Geometry check sheet. Reference: the model listing, model coordinates, mm. A direction names the side the tool comes from. Round coordinates to 2 decimals unless told otherwise and drop trailing zeros. Write each loop counter-clockwise with the first axis right and the second up, starting at its lowest first coordinate (ties: lowest second). Pieces come first, ordered by that corner, then holes. Notation, with made-up numbers: M 81,35.25 L 85,35.25 A18 ccw 85,58.25 Z; hole C 10.5,-11.75 d5. An arc over 180 degrees is marked long. Use a Markdown table: item, result.
```python
from build123d import *

# Parameters (mm, degrees)
CYLINDER052_R             = 6.25
CYLINDER052_DEPTH         = 17
CYLINDER051_R             = 2.1
CYLINDER051_DEPTH         = 10
EXTRUDE014_DEPTH          = 10
EXTRUDE016_DEPTH          = 14
EXTRUDE015_DEPTH          = 4
BOX021_W                  = 47
BOX021_H                  = 26
BOX021_DEPTH              = 4
CYLINDER044_R             = 4
CYLINDER044_DEPTH         = 4
BOX014_W                  = 13
BOX014_H                  = 8
BOX014_DEPTH              = 4
FUSION015_PLACEMENT_ANGLE = 180
CYLINDER039_R             = 1.6
CYLINDER039_DEPTH         = 15
CYLINDER043_R             = 3.7
CYLINDER043_DEPTH         = 10
CYLINDER045_R             = 7.5
CYLINDER045_DEPTH         = 6
CYLINDER042_R             = 9.6
CYLINDER042_DEPTH         = 6
BOX012_W                  = 26
BOX012_H                  = 42
BOX012_DEPTH              = 1
BOX013_W                  = 47
BOX013_H                  = 10
BOX013_DEPTH              = 37


with BuildPart() as cylinder052:
    # Cylinder052 → Cylinder052 (new body)
    with BuildSketch(Plane.XY.offset(10)):
        Circle(CYLINDER052_R)
    extrude(amount=CYLINDER052_DEPTH)


with BuildPart() as fusion022:
    # Cylinder051 → Cylinder051 (new body)
    with BuildSketch(Plane.XY):
        Circle(CYLINDER051_R)
    extrude(amount=CYLINDER051_DEPTH)

    # Fusion022: union Cylinder052
    add(cylinder052.part)


with BuildPart() as fusion022_1:
    # Fusion022 placement: moved
    add(fusion022.part.moved(Location((12, 12, -6))))


with BuildPart() as extrude014:
    # Sketch010 → Extrude014 (new body)
    with BuildSketch(Plane.XY):
        with BuildLine():
            ThreePointArc((35.736492, 10), (36.2, 15), (35.736492, 20))
            ThreePointArc((35.736492, 20), (33.490746, 22.111711), (31.244999, 20))
            ThreePointArc((31.244999, 10), (31.8, 15), (31.244999, 20))
            ThreePointArc((31.244999, 10), (33.490746, 7.888289), (35.736492, 10))
        make_face()
    extrude(amount=-EXTRUDE014_DEPTH)


with BuildPart() as extrude014_1:
    # Extrude014 placement: moved
    add(extrude014.part.moved(Location((2, -3, 8))))


with BuildPart() as extrude016:
    # Sketch015 → Extrude016 (new body)
    with BuildSketch(Plane.YZ):
        Polygon((0, 4), (26, 4), (26, 23), align=None)
    extrude(amount=EXTRUDE016_DEPTH)


with BuildPart() as extrude015:
    # Sketch014 → Extrude015 (new body)
    with BuildSketch(Plane.YZ):
        Polygon((0, 4), (26, 4), (26, 37), align=None)
    extrude(amount=EXTRUDE015_DEPTH)


with BuildPart() as extrude015_1:
    # Extrude015 placement: moved
    add(extrude015.part.moved(Location((43, 0, 0))))


with BuildPart() as box021:
    # Box021 → Box021 (new body)
    with BuildSketch(Plane.XY):
        with Locations((23.5, 13)):
            Rectangle(BOX021_W, BOX021_H)
    extrude(amount=BOX021_DEPTH)


with BuildPart() as cylinder044:
    # Cylinder044 → Cylinder044 (new body)
    with BuildSketch(Plane(origin=(9, 11, -8), x_dir=(1, 0, 0), z_dir=(0, 0, 1))):
        Circle(CYLINDER044_R)
    extrude(amount=CYLINDER044_DEPTH)


with BuildPart() as fusion015:
    # Box014 → Box014 (new body)
    with BuildSketch(Plane(origin=(9, 7, -8), x_dir=(1, 0, 0), z_dir=(0, 0, 1))):
        with Locations((6.5, 4)):
            Rectangle(BOX014_W, BOX014_H)
    extrude(amount=BOX014_DEPTH)

    # Fusion015: union Cylinder044
    add(cylinder044.part)


with BuildPart() as fusion015_1:
    # Fusion015 placement: moved
    add(fusion015.part.moved(Location((13, 42, 21))).rotate(Axis((13, 42, 21), (0, 0, 1)), FUSION015_PLACEMENT_ANGLE))


with BuildPart() as cylinder039:
    # Cylinder039 → Cylinder039 (new body)
    with BuildSketch(Plane.XY):
        Circle(CYLINDER039_R)
    extrude(amount=CYLINDER039_DEPTH)


with BuildPart() as fusion016:
    # Cone002 → Cone002 (revolve)
    with BuildSketch(Plane(origin=(0, 0, 15), x_dir=(1, 0, 0), z_dir=(0, -1, 0))):
        Polygon((0, 0), (1.6, 0), (3, 3.5), (0, 3.5), align=None)
    revolve(axis=Axis((0, 0, 15), (0, 0, 1)))

    # Fusion016: union Cylinder039
    add(cylinder039.part)


with BuildPart() as fusion016_1:
    # Fusion016 placement: moved
    add(fusion016.part.moved(Location((4, 31, 13.5))))


with BuildPart() as cylinder043:
    # Cylinder043 → Cylinder043 (new body)
    with BuildSketch(Plane(origin=(4, 31, 32), x_dir=(1, 0, 0), z_dir=(0, 0, 1))):
        Circle(CYLINDER043_R)
    extrude(amount=CYLINDER043_DEPTH)


with BuildPart() as cylinder045:
    # Cylinder045 → Cylinder045 (new body)
    with BuildSketch(Plane(origin=(23.5, 30, 23.5), x_dir=(1, 0, 0), z_dir=(0, 1, 0))):
        Circle(CYLINDER045_R)
    extrude(amount=CYLINDER045_DEPTH)


with BuildPart() as cylinder042:
    # Cylinder042 → Cylinder042 (new body)
    with BuildSketch(Plane(origin=(23.5, 26, 23.5), x_dir=(1, 0, 0), z_dir=(0, 1, 0))):
        Circle(CYLINDER042_R)
    extrude(amount=CYLINDER042_DEPTH)


with BuildPart() as box012:
    # Box012 → Box012 (new body)
    with BuildSketch(Plane(origin=(-4, 13, 23), x_dir=(1, 0, 0), z_dir=(0, 0, 1))):
        with Locations((13, 21)):
            Rectangle(BOX012_W, BOX012_H)
    extrude(amount=BOX012_DEPTH)


with BuildPart() as cut054:
    # Box013 → Box013 (new body)
    with BuildSketch(Plane(origin=(0, 26, 0), x_dir=(1, 0, 0), z_dir=(0, 0, 1))):
        with Locations((23.5, 5)):
            Rectangle(BOX013_W, BOX013_H)
    extrude(amount=BOX013_DEPTH)

    # Cut047: cut Box012
    add(box012.part, mode=Mode.SUBTRACT)

    # Cut048: cut Cylinder042
    add(cylinder042.part, mode=Mode.SUBTRACT)

    # Cut049: cut Cylinder045
    add(cylinder045.part, mode=Mode.SUBTRACT)

    # Cut050: cut Cylinder043
    add(cylinder043.part, mode=Mode.SUBTRACT)

    # Cut051: cut Fusion016
    add(fusion016_1.part, mode=Mode.SUBTRACT)

    # Cut052: cut Fusion015
    add(fusion015_1.part, mode=Mode.SUBTRACT)

    # Fusion023: union Box021
    add(box021.part)

    # Fusion024: union Extrude016, Extrude015
    add(extrude016.part)
    add(extrude015_1.part)

    # Cut053: cut Extrude014
    add(extrude014_1.part, mode=Mode.SUBTRACT)

    # Cut054: cut Fusion022
    add(fusion022_1.part, mode=Mode.SUBTRACT)


with BuildPart() as cut054_1:
    # Cut054 placement: moved
    add(cut054.part.moved(Location((19, 198, -23))))


solid = cut054_1.part
```
Item 1: Access from +Z, -Z, +X, -X, +Y, -Y to the whole of each face (thin tool, end or side, straight path). Record for faces 5 (the face through (22.792, 230.586, -3.042)), 6 (the face through (21, 229, -6)), 7 (the face through (24.35, 211.18, -9.37)), 8 (the face through (54.44, 202.89, -20.97)).
Outcome:
| item | result |
|---|---|
| face 5 | +Z |
| face 6 | -X |
| face 7 | +Z, -X, -Y |
| face 8 | +Z, -Z |
Item 2: Material ranges on line 1 along X through (y, z) = (210, -20); line 2 along Y through (x, z) = (23, 12.95); line 3 along Y through (x, z) = (23, 2.15), recorded low to high. Write a range as from..to.
Outcome:
| item | result |
|---|---|
| line 1 | x = 19..28.9, 33.1..52.8, 57.2..66 |
| line 2 | y = 224..225.3, 232.7..234 |
| line 3 | y = 224..227.4, 230.6..234 |
Item 3: Cross-section at A-A, the plane y = 229. Record the cut outline in (x, z).
Outcome:
| item | result |
|---|---|
| outline | M 19,-23 L 66,-23 L 66,14 L 26.7,14 L 26.7,9 L 26,9 L 24.6,5.5 L 24.6,1 L 32.91,1 A9.6 cw long 32.91,0 L 24.6,0 L 24.6,-6 L 27,-6 L 27,-10 L 19,-10 Z; M 19,-6 L 21.4,-6 L 21.4,0 L 19,0 Z; M 19,1 L 21.4,1 L 21.4,5.5 L 20,9 L 19.3,9 L 19.3,14 L 19,14 Z |
Item 4: Mould release check, pull along Z, two halves, no side actions. Record for faces 1 (the face through (42, 234, -9)), 2 (the face through (21, 225, -8)), 3 (the face through (21, 233, -8)), 4 (the face through (63.97, 211.18, -2.27)): +Z half, -Z half, draft (parallel to the pull), parting line (faces both ways), or undercut.
Outcome:
| item | result |
|---|---|
| face 1 | draft |
| face 2 | undercut |
| face 3 | undercut |
| face 4 | +Z half |
Item 5: Cross-section at C-C, the plane x = 42.5. Record the cut outline in (y, z), and give its area (3 significant figures).
Outcome:
| item | result |
|---|---|
| outline | M 198,-23 L 234,-23 L 234,-7 L 230,-7 L 230,-9.1 L 224,-9.1 L 224,-19 L 198,-19 Z; M 224,10.1 L 230,10.1 L 230,8 L 234,8 L 234,14 L 224,14 Z |
| area | 299 mm2 |
Item 6: Cross-section at D-D, the plane x = 30.5. Record the cut outline in (y, z).
Outcome:
| item | result |
|---|---|
| outline | M 198,-23 L 207.96,-23 L 207.96,-19 L 203.77,-19 L 203.77,-14.78 L 198,-19 Z; M 212.04,-23 L 234,-23 L 234,0 L 224,0 L 216.23,-5.68 L 216.23,-19 L 212.04,-19 Z; M 224,1 L 234,1 L 234,14 L 224,14 Z |
Item 7: Cross-section at B-B, the plane z = 3. Record the cut outline in (x, y).
Outcome:
| item | result |
|---|---|
| outline | M 19,224 L 33.23,224 L 33.23,230 L 35.43,230 L 35.43,234 L 19,234 Z; M 49.57,230 L 51.77,230 L 51.77,224 L 62,224 L 62,215.33 L 66,215.33 L 66,234 L 49.57,234 Z; hole C 23,229 d3.2 |
Item 8: Go/stop test with flat-tipped pins: pin 1 (4.5 mm diameter, centred on x = 23, y = 229, fed in from +Z) (3 decimals); pin 2 (3 mm diameter, centred on x = 54.5, y = 202.5, fed in from +Z); pin 3 (2.5 mm diameter, centred on x = 23, y = 229, fed in from +Z); pin 4 (2 mm diameter, centred on x = 38, z = -3, fed in from -Y). Record where each tip stops, or that it passes through.
Outcome:
| item | result |
|---|---|
| pin 1 | stops at z = 7.125 |
| pin 2 | stops at z = -19 |
| pin 3 | stops at z = -10 |
| pin 4 | passes through |
